```python
from build123d import *

# Parameters (mm, degrees)
CROQUIS1_R              = 3
SALIENTE_EXTRUIR1_DEPTH = 4
CORTAR_EXTRUIR1_DEPTH   = 2
CROQUIS3_R              = 1.7
CORTAR_EXTRUIR2_DEPTH   = 10


with BuildPart() as part:
    # Croquis1 → Saliente-Extruir1 (new body)
    with BuildSketch(Plane.XY):
        with BuildLine():
            Line((-7.200520814, 3.25), (-15, 3.25))
            Line((-15, 3.25), (-15, -3.25))
            Line((-15, -3.25), (-7.200520814, -3.25))
            ThreePointArc((-7.200520814, -3.25), (0, -7.9), (7.200520814, -3.25))
            Line((7.200520814, -3.25), (15, -3.25))
            Line((15, -3.25), (15, 3.25))
            Line((15, 3.25), (7.200520814, 3.25))
            ThreePointArc((7.200520814, 3.25), (0, 7.9), (-7.200520814, 3.25))
        make_face()
        Circle(CROQUIS1_R, mode=Mode.SUBTRACT)
    extrude(amount=SALIENTE_EXTRUIR1_DEPTH)

    # Croquis2 → Cortar-Extruir1 (cut)
    with BuildSketch(Plane.XY.offset(4)):
        Polygon((-14.35, 0), (-12.675, -2.901185103), (-9.325, -2.901185103), (-7.65, 0), (-9.325, 2.901185103), (-12.675, 2.901185103), align=None)
        Polygon((14.35, 0), (12.675, 2.901185103), (9.325, 2.901185103), (7.65, 0), (9.325, -2.901185103), (12.675, -2.901185103), align=None)
    extrude(amount=-CORTAR_EXTRUIR1_DEPTH, mode=Mode.SUBTRACT)

    # Croquis3 → Cortar-Extruir2 (cut)
    with BuildSketch(Plane.XY.offset(4)):
        with Locations((-11, 0)):
            Circle(CROQUIS3_R)
        with Locations((11, 0)):
            Circle(CROQUIS3_R)
    extrude(amount=-CORTAR_EXTRUIR2_DEPTH, mode=Mode.SUBTRACT)


solid = part.part
```
Part model, mm, in its own coordinate system. A direction names the side the tool comes from. Coordinates: 2 decimals unless noted, no trailing zeros. Write each loop counter-clockwise with the first axis right and the second up, starting at its lowest first coordinate (ties: lowest second). Pieces come first, ordered by that corner, then holes.
Item 1: Pin check, flat tips, straight feed: pin 1 (0.6 mm diameter, centred on x = 10.5, z = 2.5, fed in from +Y); pin 2 (1 mm diameter, centred on x = 5, z = 2, fed in from +Y); pin 3 (6.5 mm diameter, centred on x = 12, y = 1, fed in from +Z); pin 4 (2 mm diameter, centred on x = 11, y = 0, fed in from +Z). Stop position of each tip, or through.
Item 2: Slice it at B-B (x = -11). Write the cut outline in (y, z).
Item 3: Which spindle directions (+Z, -Z, +X, -X, +Y, -Y) get a long thin tool onto all of the face, cutting with end or side? Do faces 1 (the face through (11, -3.25, 2)), 2 (the face through (11, 2.901, 3)), 3 (the face through (-9.43, -0.65, 1.01)). Say none if no direction does.
Item 4: Slice it at C-C (x = 0). Write the cut outline in (y, z).
Item 5: Probe line 1 (Y direction, x = -11, z = 0.9); line 2 (Y direction, x = 0, z = 1.8); line 3 (X direction, y = -2, z = 3.65). List the from-to ranges inside material, lowest first.
Item 6: Slice it at A-A (z = 1.7). Write the cut outline in (x, y).
Item 7: Mould opens along Y. For faces 4 (the face through (8.476, -1.43, 3.014)), 5 (the face through (-11, -3.25, 2)), 6 (the face through (0.1, 7.9, 2)) say: released by +Y, released by -Y, zero draft, split by the parting line, or undercut.
Item 8: Slice it at D-D (y = 6.75). Write the cut outline in (x, z), and give its area (3 significant figures).
Results found:
1. pin 1: stops at y = 3.25
1. pin 2: stops at y = 6.49
1. pin 3: stops at z = 4
1. pin 4: passes through
2. outline: (-3.25, 0) - (-1.7, 0) - (-1.7, 2) - (-2.9, 2) - (-2.9, 4) - (-3.25, 4) - close; (1.7, 0) - (3.25, 0) - (3.25, 4) - (2.9, 4) - (2.9, 2) - (1.7, 2) - close
3. face 1: +Z, -Z, +X, -Y
3. face 2: +Z
3. face 3: +Z, -Z
4. outline: (-7.9, 0) - (-3, 0) - (-3, 4) - (-7.9, 4) - close; (3, 0) - (7.9, 0) - (7.9, 4) - (3, 4) - close
5. line 1: y = -3.25 to -1.7, 1.7 to 3.25
5. line 2: y = -7.9 to -3, 3 to 7.9
5. line 3: x = -15 to -13.2, -8.8 to -2.24, 2.24 to 8.8, 13.2 to 15
6. outline: (-15, -3.25) - (-7.2, -3.25) arc R7.9 ccw to (7.2, -3.25) - (15, -3.25) - (15, 3.25) - (7.2, 3.25) arc R7.9 ccw to (-7.2, 3.25) - (-15, 3.25) - close; hole circle Ø3.4 at (-11, 0); hole circle Ø6 at (0, 0); hole circle Ø3.4 at (11, 0)
7. face 4: undercut
7. face 5: released by -Y
7. face 6: released by +Y
8. outline: (-4.1, 0) - (4.1, 0) - (4.1, 4) - (-4.1, 4) - close
8. area: 32.8 mm2
